Answer from the drawing. Dimensions are ordinates in mm from the lowest x, y and z of the part. A direction names the side the tool comes from. Give positions to 0.01 mm unless a question says otherwise; leave off trailing zeros. Order: outer loops, then holes, each group sorted by start corner. A loop starts at its lowest first (then second) coordinate and runs counter-clockwise, first axis right, second up. Notation, with made-up numbers: (-23, 70) - (14, 70) arc R36 cw to (14, 105) - close; hole circle Ø9 at (42, 11). An arc over 180 degrees is marked (long way). Write each question's results on one line, items separated by ' | '.
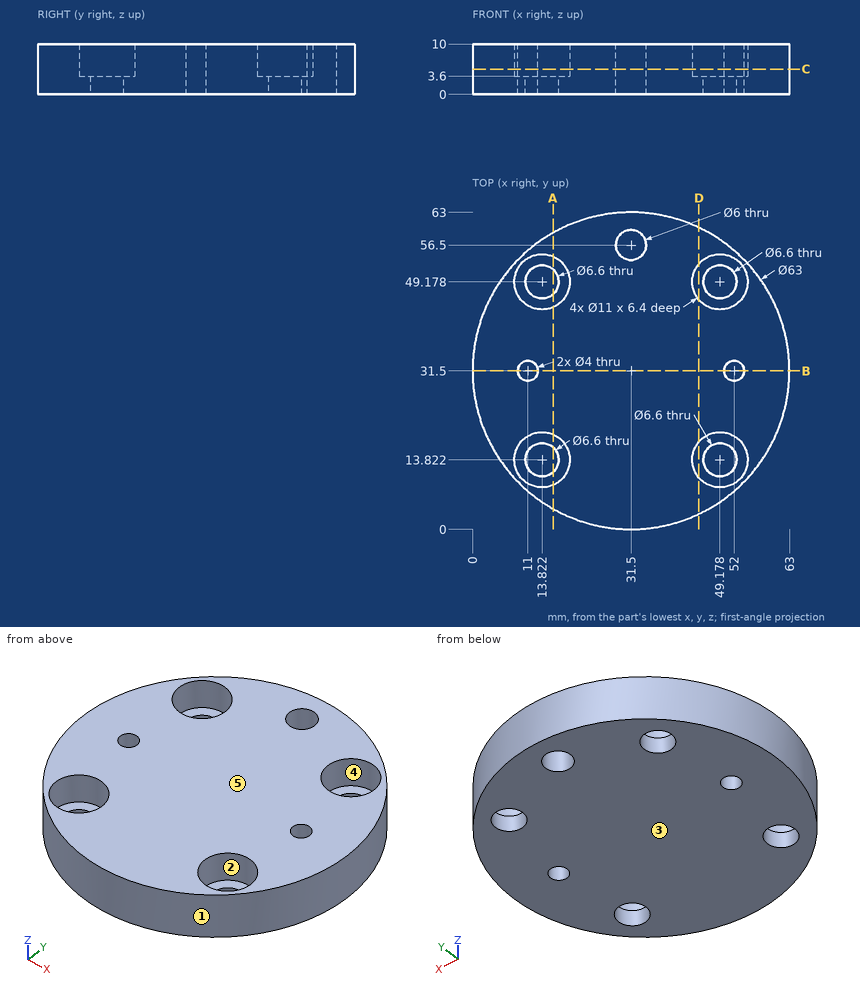
(1) Section B-B (y = 31.5) is taken. Give the vertices of the cut face in (x, z), plus the area to 3 significant figures.
Conclusion:
outline: (0, 0) - (9, 0) - (9, 10) - (0, 10) - close; (13, 0) - (50, 0) - (50, 10) - (13, 10) - close; (54, 0) - (63, 0) - (63, 10) - (54, 10) - close | area: 550 mm^2
(2) Section C-C (z = 5) is taken. Give the vertices of the cut face in (x, y).
Conclusion:
outline: circle Ø63 at (31.5, 31.5); hole circle Ø11 at (13.82, 13.82); hole circle Ø11 at (13.82, 49.18); hole circle Ø4 at (11, 31.5); hole circle Ø6 at (31.5, 56.5); hole circle Ø11 at (49.18, 13.82); hole circle Ø11 at (49.18, 49.18); hole circle Ø4 at (52, 31.5)
(3) For the marked faces 4 and 5, determine the directions among +Z, -Z, +X, -X, +Y, -Y from which every point of the face is accessible in a straight line to the end or side of a thin tool.
Conclusion:
face 4: +Z | face 5: +Z, +X, -X, +Y, -Y
(4) Section D-D (x = 45) is taken. Give the vertices of the cut face in (y, z) (1 decimal), plus the area to 3 significant figures.
Conclusion:
outline: (3, 0) - (60, 0) - (60, 10) - (52.8, 10) - (52.8, 3.6) - (45.6, 3.6) - (45.6, 10) - (17.4, 10) - (17.4, 3.6) - (10.2, 3.6) - (10.2, 10) - (3, 10) - close | area: 478 mm^2
(5) Section A-A (x = 16) is taken. Give the vertices of the cut face in (y, z).
Conclusion:
outline: (4.08, 0) - (11.34, 0) - (11.34, 3.6) - (8.77, 3.6) - (8.77, 10) - (4.08, 10) - close; (16.3, 0) - (46.7, 0) - (46.7, 3.6) - (44.13, 3.6) - (44.13, 10) - (18.87, 10) - (18.87, 3.6) - (16.3, 3.6) - close; (51.66, 0) - (58.92, 0) - (58.92, 10) - (54.23, 10) - (54.23, 3.6) - (51.66, 3.6) - close
(6) Each of these flat-tipped pins is pushed along its axis until it touches: pin 1 (4 mm diameter, centred on x = 7.5, z = 5.5, fed in from -Y) (1 decimal); pin 2 (3.5 mm diameter, centred on x = 51.5, y = 12, fed in from +Z); pin 3 (4 mm diameter, centred on x = 11, z = 5, fed in from -Y) (1 decimal). Where does it stop, or does it pass through?
Conclusion:
pin 1: y = 9 | pin 2: z = 3.6 | pin 3: y = 6
(7) Consider probe 1 along X at (y, z) = (31, 2.5); probe 2 along Y at (x, z) = (53, 7.25); probe 3 along Y at (x, z) = (14, 4.25) (1 decimal). Determine where each line is inside the solid, lowest interval first. Write a range as [from, to].
Conclusion:
probe 1: [0, 9.06], [12.94, 50.06], [53.94, 63] | probe 2: [8.48, 9.87], [17.78, 29.77], [33.23, 45.22], [53.13, 54.52] | probe 3: [5.3, 8.3], [19.3, 43.7], [54.7, 57.7]
(8) The mould has two halves that part along X. Classify the marked faces 1, 2 and 3: pulls with the +X half, pulls with the -X half, needs draft (parallel to the pull), parting line crosses it, or undercut.
Conclusion:
face 1: parting line crosses it | face 2: undercut | face 3: needs draft
